from build123d import *

# Parameters (mm, degrees)
ESQUISSE1_R      = 4
EXTRUSION1_DEPTH = 150
CHANFREIN1_SIZE  = 0.5
ESQUISSE2_R      = 2.5
EXTRUSION2_DEPTH = 15
ESQUISSE3_R      = 2.5
EXTRUSION3_DEPTH = 15


with BuildPart() as part:
    # Esquisse1 → Extrusion1 (new body)
    with BuildSketch(Plane(origin=(0, 0, 0), x_dir=(1, 0, 0), z_dir=(0, 1, 0))):
        Circle(ESQUISSE1_R)
    extrude(amount=EXTRUSION1_DEPTH)

    # Chanfrein1
    chanfrein1_edges = [part.edges().sort_by_distance(p)[0] for p in [
        (-4, 0, 0),
        (-4, 150, 0),
    ]]
    chamfer(chanfrein1_edges, length=CHANFREIN1_SIZE)

    # Esquisse2 → Extrusion2 (cut)
    with BuildSketch(Plane.XZ):
        Circle(ESQUISSE2_R)
    extrude(amount=-EXTRUSION2_DEPTH, mode=Mode.SUBTRACT)

    # Esquisse3 → Extrusion3 (cut)
    with BuildSketch(Plane(origin=(0, 150, 0), x_dir=(1, 0, 0), z_dir=(0, 1, 0))):
        Circle(ESQUISSE3_R)
    extrude(amount=-EXTRUSION3_DEPTH, mode=Mode.SUBTRACT)


solid = part.part
The model under review builds one solid part; all positions refer to its coordinate system, in mm. A direction names the side the tool comes from. Round coordinates to 2 decimals unless told otherwise and drop trailing zeros. Order: outer loops, then holes, each group sorted by start corner. A loop starts at its lowest first (then second) coordinate and runs counter-clockwise, first axis right, second up. Notation, with made-up numbers: (30.25, -30) -> (37.25, -30) arc R12 ccw to (37.25, -20) -> close; hole circle Ø10 at (18.25, 80). An arc over 180 degrees is marked (long way). Return JSON: item names as keys, results as strings.
1. For L1, parallel to Z at x = 0, y = 12; L2, parallel to Y at x = -0.25, z = 0, list the stretches that pass through material, from the lowest coordinate up. Write a range as [from, to].
Answer block:
{"L1": "z = [-4, -2.5], [2.5, 4]", "L2": "y = [15, 135]"}
2. Take a section at C-C (y = 11.5). Write out the cut boundary in (x, z), then the cut area to 3 significant figures.
Answer block:
{"outline": "circle Ø8 at (0, 0); hole circle Ø5 at (0, 0)", "area": "30.6 mm²"}
3. Take a section at D-D (y = 122.5). Write out the cut boundary in (x, z).
Answer block:
{"outline": "circle Ø8 at (0, 0)"}
4. Insertion check: P1, Ø2.5, axis at x = -0.5, z = 0.5, coming from the -Y side; P2, Ø2, axis at x = -2, y = 79.5, coming from the +Z side; P3, Ø2, axis at y = 89.5, z = 1.5, coming from the +X side. Each pin has a flat end and moves straight along its axis. Give the tip position at first contact, or say it passes through.
Answer block:
{"P1": "stops at y = 15", "P2": "stops at z = 3.87", "P3": "stops at x = 3.97"}
5. Take a section at A-A (z = 0). Write out the cut boundary in (x, y), then the cut area to 3 significant figures.
Answer block:
{"outline": "(-4, 0.5) -> (-3.5, 0) -> (-2.5, 0) -> (-2.5, 15) -> (2.5, 15) -> (2.5, 0) -> (3.5, 0) -> (4, 0.5) -> (4, 149.5) -> (3.5, 150) -> (2.5, 150) -> (2.5, 135) -> (-2.5, 135) -> (-2.5, 150) -> (-3.5, 150) -> (-4, 149.5) -> close", "area": "1,050 mm²"}
6. Take a section at B-B (x = 0). Write out the cut boundary in (y, z), then the cut area to 3 significant figures.
Answer block:
{"outline": "(0, -3.5) -> (0.5, -4) -> (149.5, -4) -> (150, -3.5) -> (150, -2.5) -> (135, -2.5) -> (135, 2.5) -> (150, 2.5) -> (150, 3.5) -> (149.5, 4) -> (0.5, 4) -> (0, 3.5) -> (0, 2.5) -> (15, 2.5) -> (15, -2.5) -> (0, -2.5) -> close", "area": "1,050 mm²"}
7. For faces 4 (the face through (2, 0, 2)), 5 (the face through (-0.54, 142.6, 2.44)), 6 (the face through (0, 15, 0)), list the 3-axis set-ups (+Z, -Z, +X, -X, +Y, -Y) from which the entire face can be reached by the end or side of a thin tool; tool diameter is ignored.
Answer block:
{"face 4": "+Z, -Z, +X, -X, -Y", "face 5": "+Y", "face 6": "-Y"}
8. The part is to be moulded in two halves that separate along Z. For faces 1 (the face through (2, 150, 2)), 2 (the face through (-0.54, 7.4, -2.44)), 3 (the face through (-0.867, 73.957, 3.905)), say which applies: +Z half, -Z half, draft (parallel to the pull), parting line (faces both ways), or undercut.
Answer block:
{"face 1": "draft", "face 2": "undercut", "face 3": "parting line"}
